Read the model definition and answer for the solid it produces. Units are mm, in the model's axes. A direction names the side the tool comes from. Give positions to 0.01 mm unless a question says otherwise; leave off trailing zeros. Write each loop counter-clockwise with the first axis right and the second up, starting at its lowest first coordinate (ties: lowest second). Pieces come first, ordered by that corner, then holes. Notation, with made-up numbers: (80.5, 57.25) -> (87.5, 57.25) arc R16 cw to (87.5, 74.25) -> close; hole circle Ø8 at (20.5, 61.5). An arc over 180 degrees is marked (long way). Put each result on its own line as item: value. Start each with the question number.
from build123d import *

# Parameters (mm, degrees)
ESBO_O1_R                  = 17.5
ESBO_O1_R_2                = 6.75
RESSALTO_EXTRUS_O1_DEPTH   = 10
ESBO_O2_R                  = 3
ESBO_O2_R_2                = 1.5
CORTE_EXTRUS_O1_DEPTH      = 6
CORTE_EXTRUS_O2_REACH      = 42.389
CORTE_EXTRUS_O2_END_RADIUS = 6.75
ESBO_O2_3_R                = 1.5
PADR_OCIRCULAR1_COUNT      = 4
ESBO_O5_R                  = 1.5
CORTE_EXTRUS_O3_DEPTH      = 5
PADR_OCIRCULAR2_COUNT      = 4
CORTE_EXTRUS_O4_DEPTH      = 7.75
PADR_OCIRCULAR3_COUNT      = 4


with BuildPart() as part:
    # Esbo_o1 → Ressalto-extrus_o1 (new body)
    with BuildSketch(Plane.XY):
        Circle(ESBO_O1_R)
        Circle(ESBO_O1_R_2, mode=Mode.SUBTRACT)
    extrude(amount=RESSALTO_EXTRUS_O1_DEPTH)

    # Esbo_o2 → Corte-extrus_o1 (cut)
    # profile 1 of 2: a face of its own
    with BuildSketch(Plane(origin=(0, 17.5, 0), x_dir=(1, 0, 0), z_dir=(0, 1, 0))):
        with Locations(Location((0, -5, 0), (0, 0, 270))):
            Circle(ESBO_O2_R)
        with Locations((0, -5)):
            Circle(ESBO_O2_R_2, mode=Mode.SUBTRACT)
    # profile 2 of 2: a face of its own
    with BuildSketch(Plane(origin=(0, 17.5, 0), x_dir=(1, 0, 0), z_dir=(0, 1, 0))):
        with Locations((0, -5)):
            Circle(ESBO_O2_R_2)
    corte_extrus_o1 = extrude(amount=-CORTE_EXTRUS_O1_DEPTH, mode=Mode.SUBTRACT)

    # Corte-extrus_o2: up to this cylinder (the profile starts outside it)
    corte_extrus_o2_end = Plane(origin=(0, 0, 5), z_dir=(0, 0, -1)) * Cylinder(CORTE_EXTRUS_O2_END_RADIUS, 99.278, mode=Mode.PRIVATE)
    # Esbo_o2_3 → Corte-extrus_o2 (cut, up to the surface)
    with BuildSketch(Plane(origin=(0, 17.5, 0), x_dir=(1, 0, 0), z_dir=(0, 1, 0)), mode=Mode.PRIVATE) as corte_extrus_o2_sk1:
        with Locations(Location((0, -5, 0), (0, 0, 270))):
            Circle(ESBO_O2_3_R)
    corte_extrus_o2_tool1 = extrude(corte_extrus_o2_sk1.sketch, amount=-CORTE_EXTRUS_O2_REACH, mode=Mode.PRIVATE) - corte_extrus_o2_end
    corte_extrus_o2 = corte_extrus_o2_tool1.solids().sort_by_distance((0, 17.5, 5))[0]
    add(corte_extrus_o2, mode=Mode.SUBTRACT)

    # Padr_oCircular1: Corte-extrus_o1, Corte-extrus_o2 ×4 about axis
    padr_ocircular1_axis = Axis((0, 0, 0), (0, 0, 1))
    add([corte_extrus_o1.rotate(padr_ocircular1_axis, i * 360 / PADR_OCIRCULAR1_COUNT) for i in range(1, PADR_OCIRCULAR1_COUNT)], mode=Mode.SUBTRACT)
    add([corte_extrus_o2.rotate(padr_ocircular1_axis, i * 360 / PADR_OCIRCULAR1_COUNT) for i in range(1, PADR_OCIRCULAR1_COUNT)], mode=Mode.SUBTRACT)

    # Esbo_o5 → Corte-extrus_o3 (cut)
    with BuildSketch(Plane(origin=(-12.374368671, 12.374368671, 0), x_dir=(0, 0, -1), z_dir=(-0.7071067811865488, 0.7071067811865464, 0))):
        with Locations(Location((-5, 0, 0), (0, 0, 90))):
            Circle(ESBO_O5_R)
    corte_extrus_o3 = extrude(amount=-CORTE_EXTRUS_O3_DEPTH, mode=Mode.SUBTRACT)

    # Padr_oCircular2: Corte-extrus_o3 ×4 about axis
    padr_ocircular2_axis = Axis((0, 0, 0), (0, 0, 1))
    for i in range(1, PADR_OCIRCULAR2_COUNT):
        add(corte_extrus_o3.rotate(padr_ocircular2_axis, i * 360 / PADR_OCIRCULAR2_COUNT), mode=Mode.SUBTRACT)

    # Esbo_o6 → Corte-extrus_o4 (cut)
    with BuildSketch(Plane(origin=(0, 0, 0), x_dir=(-1, 0, 0), z_dir=(0, 0, -1))):
        Polygon((-11.313708499, 7.778174593), (-7.778174593, 11.313708499), (-5.656854249, 9.192388155), (-9.192388155, 5.656854249), align=None)
    corte_extrus_o4 = extrude(amount=-CORTE_EXTRUS_O4_DEPTH, mode=Mode.SUBTRACT)

    # Padr_oCircular3: Corte-extrus_o4 ×4 about axis
    padr_ocircular3_axis = Axis((0, 0, 0), (0, 0, 1))
    for i in range(1, PADR_OCIRCULAR3_COUNT):
        add(corte_extrus_o4.rotate(padr_ocircular3_axis, i * 360 / PADR_OCIRCULAR3_COUNT), mode=Mode.SUBTRACT)


solid = part.part
1) For faces 5 (the face through (-14.5, -1.8, 2.6)), 6 (the face through (10.268, -6.732, 3.821)), 7 (the face through (14.5, 1.8, 2.6)), 8 (the face through (-1.3, 11.5, 6.3)), determine the directions among +Z, -Z, +X, -X, +Y, -Y from which every point of the face is accessible in a straight line to the end or side of a thin tool.
2) A cutting plane is placed at C-C on z = 1.25. Give the vertices of the cut face in (x, y), and give its area (3 significant figures).
3) A cutting plane is placed at D-D on y = 14. Give the vertices of the cut face in (x, z).
4) Each of these flat-tipped pins is pushed along its axis until it touches: pin 1 Ø5 at (x, z) = (3.5, 4) entering from -Y; pin 2 Ø3 at (y, z) = (1, 5) entering from -X; pin 3 Ø3 at (x, z) = (-9.5, 6.5) entering from -Y; pin 4 Ø2.5 at (y, z) = (0, 5) entering from -X. Where does it stop, or does it pass through?
5) A cutting plane is placed at A-A on y = 0. Give the vertices of the cut face in (x, z), and give its area (4 significant figures).
6) For a pull along X with two mould halves and no side action, classify faces 1 (the face through (16.166, -6.703, 4.93)), 2 (the face through (-9.57, -9.52, 2.96)), 3 (the face through (9, -8, 7.75)), 4 (the face through (9.08, -0.45, 6.43)) as pulls with the +X half, pulls with the -X half, needs draft (parallel to the pull), parting line crosses it, or undercut.
7) Straight lines are drawn through the part: line 1 (Y direction, x = 7, z = 1.75); line 2 (Z direction, x = 10, y = 10); line 3 (Y direction, x = -9.1, z = 5). For each, find the intervals that lie inside material, in ascending order. Write a range as [from, to].
Results found:
1. face 5: -X
1. face 6: -Z
1. face 7: +X
1. face 8: +Y
2. outline: circle Ø35 at (0, 0); hole (-11.31, -7.78) -> (-7.78, -11.31) -> (-5.66, -9.19) -> (-9.19, -5.66) -> close; hole (-11.31, 7.78) -> (-9.19, 5.66) -> (-5.66, 9.19) -> (-7.78, 11.31) -> close; hole circle Ø13.5 at (0, 0); hole (5.66, -9.19) -> (7.78, -11.31) -> (11.31, -7.78) -> (9.19, -5.66) -> close; hole (5.66, 9.19) -> (9.19, 5.66) -> (11.31, 7.78) -> (7.78, 11.31) -> close
2. area: 759 mm²
3. outline: (-10.5, 0) -> (10.5, 0) -> (10.5, 10) -> (-10.5, 10) -> close; hole circle Ø6 at (0, 5)
4. pin 1: stops at y = -17.43
4. pin 2: stops at x = -11.5
4. pin 3: stops at y = -15.56
4. pin 4: passes through
5. outline: (-17.5, 0) -> (-6.75, 0) -> (-6.75, 3.5) -> (-11.5, 3.5) -> (-11.5, 2) -> (-17.5, 2) -> close; (-17.5, 8) -> (-11.5, 8) -> (-11.5, 6.5) -> (-6.75, 6.5) -> (-6.75, 10) -> (-17.5, 10) -> close; (6.75, 0) -> (17.5, 0) -> (17.5, 2) -> (11.5, 2) -> (11.5, 3.5) -> (6.75, 3.5) -> close; (6.75, 6.5) -> (11.5, 6.5) -> (11.5, 8) -> (17.5, 8) -> (17.5, 10) -> (6.75, 10) -> close
5. area: 114.5 mm²
6. face 1: parting line crosses it
6. face 2: undercut
6. face 3: undercut
6. face 4: needs draft
7. line 1: y = [-16.04, -10.54], [-7.85, 7.85], [10.54, 16.04]
7. line 2: z = [0, 3.5], [6.5, 10]
7. line 3: y = [-14.95, -11.22], [-5.75, -1.5], [1.5, 5.75], [11.22, 14.95]
